Part model, mm, in its own coordinate system. A direction names the side the tool comes from. Round coordinates to 2 decimals unless told otherwise and drop trailing zeros. Loops run counter-clockwise (first coordinate to the right, second up) from the corner with the lowest first, then second, coordinate; pieces in that order, holes last.
(1) Probe probe 1 along Y at (x, z) = (45, 17.5); probe 2 along X at (y, z) = (-1.5, 6); probe 3 along Y at (x, z) = (49.4, 140). List the from-to ranges inside material, lowest first.
(2) Cut at D-D on y = -9. List the corners of the cut face in (x, z).
(3) Cut at C-C on y = -20. List the corners of the cut face in (x, z), then the cut area to 3 significant figures.
(4) Tool access for faces 1 (the face through (0, -8, 74)), 2 (the face through (1, -8, 74)): list every direction of +Z, -Z, +X, -X, +Y, -Y with a clear straight run to the whole face (end or side of a thin tool).
(5) Cut at A-A on x = 27. List the corners of the cut face in (y, z).
(6) Cut at B-B on z = 140. List the corners of the cut face in (x, y).
(7) Mould opens along Y. For faces 3 (the face through (25, -32.083, 74)), 4 (the face through (0.8, 3.1, 0)), 5 (the face through (25, 16.917, 74)) say: +Y half, -Y half, draft (parallel to the pull), parting line (faces both ways), or undercut.
from build123d import *

# Parameters (mm, degrees)
F0_W     = 50
F0_H     = 50
F0_W_2   = 48
F0_H_2   = 48
F1_DEPTH = 150
F2_R     = 2.5
F3_DEPTH = 50


with BuildPart() as f1:
    # F0 (on Top) → F1 (new body)
    with BuildSketch(Plane.XY):
        with Locations((25, -8.0827108582)):
            Rectangle(F0_W, F0_H)
        with Locations((25, -8.0827108582)):
            Rectangle(F0_W_2, F0_H_2, mode=Mode.SUBTRACT)
    extrude(amount=F1_DEPTH)

    # F2 (on face) → F3 (cut)
    with BuildSketch(Plane.YZ.offset(50)):
        with Locations((-8.0827108582, 140)):
            Circle(F2_R)
        with BuildLine():
            Line((1.9172891418, 120), (-3.0827108582, 120))
            ThreePointArc((-3.0827108582, 120), (-1.6182447641, 116.4644660941), (1.9172891418, 115))
            Line((1.9172891418, 115), (1.9172891418, 120))
        make_face()
        with BuildLine():
            ThreePointArc((6.9172891418, 120), (1.9172891418, 125), (-3.0827108582, 120))
            Line((-3.0827108582, 120), (1.9172891418, 120))
            Line((1.9172891418, 120), (1.9172891418, 115))
            ThreePointArc((1.9172891418, 115), (5.4528230478, 116.4644660941), (6.9172891418, 120))
        make_face()
        with BuildLine():
            ThreePointArc((-13.0827108582, 100), (-14.5471769522, 103.5355339059), (-18.0827108582, 105))
            Line((-18.0827108582, 105), (-18.0827108582, 100))
            Line((-18.0827108582, 100), (-13.0827108582, 100))
        make_face()
        with BuildLine():
            Line((-18.0827108582, 100), (-18.0827108582, 105))
            ThreePointArc((-18.0827108582, 105), (-21.6182447641, 96.4644660941), (-13.0827108582, 100))
            Line((-13.0827108582, 100), (-18.0827108582, 100))
        make_face()
        with BuildLine():
            Line((1.9172891418, 100), (1.9172891418, 105))
            ThreePointArc((1.9172891418, 105), (-1.6182447641, 103.5355339059), (-3.0827108582, 100))
            Line((-3.0827108582, 100), (1.9172891418, 100))
        make_face()
        with BuildLine():
            ThreePointArc((6.9172891418, 100), (5.4528230478, 103.5355339059), (1.9172891418, 105))
            Line((1.9172891418, 105), (1.9172891418, 100))
            Line((1.9172891418, 100), (-3.0827108582, 100))
            ThreePointArc((-3.0827108582, 100), (1.9172891418, 95), (6.9172891418, 100))
        make_face()
        with BuildLine():
            Line((-18.0827108582, 120), (-18.0827108582, 125))
            ThreePointArc((-18.0827108582, 125), (-21.6182447641, 123.5355339059), (-23.0827108582, 120))
            Line((-23.0827108582, 120), (-18.0827108582, 120))
        make_face()
        with BuildLine():
            Line((-18.0827108582, 120), (-23.0827108582, 120))
            ThreePointArc((-23.0827108582, 120), (-21.6182447641, 116.4644660941), (-18.0827108582, 115))
            Line((-18.0827108582, 115), (-18.0827108582, 120))
        make_face()
        with BuildLine():
            ThreePointArc((-13.0827108582, 120), (-14.5471769522, 123.5355339059), (-18.0827108582, 125))
            Line((-18.0827108582, 125), (-18.0827108582, 120))
            Line((-18.0827108582, 120), (-13.0827108582, 120))
        make_face()
        with BuildLine():
            Line((-13.0827108582, 120), (-18.0827108582, 120))
            Line((-18.0827108582, 120), (-18.0827108582, 115))
            ThreePointArc((-18.0827108582, 115), (-14.5471769522, 116.4644660941), (-13.0827108582, 120))
        make_face()
    extrude(amount=-F3_DEPTH, mode=Mode.SUBTRACT)


solid = f1.part
Final values:
1. probe 1: y = -33.08 to -32.08, 15.92 to 16.92
1. probe 2: x = 0 to 1, 49 to 50
1. probe 3: y = -33.08 to -10.58, -5.58 to 16.92
2. outline: (0, 0) - (1, 0) - (1, 137.67) - (0, 137.67) - close; (0, 142.33) - (1, 142.33) - (1, 150) - (0, 150) - close; (49, 0) - (50, 0) - (50, 137.67) - (49, 137.67) - close; (49, 142.33) - (50, 142.33) - (50, 150) - (49, 150) - close
3. outline: (0, 0) - (1, 0) - (1, 95.38) - (0, 95.38) - close; (0, 104.62) - (1, 104.62) - (1, 115.38) - (0, 115.38) - close; (0, 124.62) - (1, 124.62) - (1, 150) - (0, 150) - close; (49, 0) - (50, 0) - (50, 95.38) - (49, 95.38) - close; (49, 104.62) - (50, 104.62) - (50, 115.38) - (49, 115.38) - close; (49, 124.62) - (50, 124.62) - (50, 150) - (49, 150) - close
3. area: 263 mm2
4. face 1: +Z, -Z, -X, +Y, -Y
4. face 2: +Z, -Z
5. outline: (-33.08, 0) - (-32.08, 0) - (-32.08, 150) - (-33.08, 150) - close; (15.92, 0) - (16.92, 0) - (16.92, 150) - (15.92, 150) - close
6. outline: (0, -33.08) - (50, -33.08) - (50, -10.58) - (49, -10.58) - (49, -32.08) - (1, -32.08) - (1, -10.58) - (0, -10.58) - close; (0, -5.58) - (1, -5.58) - (1, 15.92) - (49, 15.92) - (49, -5.58) - (50, -5.58) - (50, 16.92) - (0, 16.92) - close
7. face 3: undercut
7. face 4: draft
7. face 5: +Y half
